Verification items for the finished model (mm, model axes). A direction names the side the tool comes from. Give positions to 0.01 mm unless a question says otherwise; leave off trailing zeros. Loops run counter-clockwise (first coordinate to the right, second up) from the corner with the lowest first, then second, coordinate; pieces in that order, holes last. Notation, with made-up numbers: (77.5, 74.5) -> (85.5, 74.5) arc R8 cw to (85.5, 81.5) -> close; hole circle Ø3 at (61.5, -12). An arc over 180 degrees is marked (long way). Answer in a Markdown table with one row per item. Add a question column.
Q1. Gauge pin test, flat ends, axial feed: P1, Ø12, axis at x = 16.5, y = 27.5, coming from the -Z side; P2, Ø1.8, axis at x = 6.5, z = 3.5, coming from the -Y side. Record the tip position at first contact, or that the pin passes through.
Q2. Material ranges on probe 1 along Y at (x, z) = (10, 4.05); probe 2 along Y at (x, z) = (12, 2.75); probe 3 along X at (y, z) = (32, 2.95), recorded low to high.
Q3. Section check C-C on y = 7. Enter the section's corners in (x, z), and give its area (3 significant figures).
Q4. Section check B-B on z = 2.5. Give the number of separate pieces and of enclosed holes in the cut face, and give its area (3 significant figures).
Q5. Section check A-A on x = 10. Enter the section's corners in (y, z).
Q6. Section check D-D on y = 18.5. Enter the section's corners in (x, z).
Q7. Release check for a two-part mould opening along Y. For faces 1 (the face through (10, 40, 2)), 2 (the face through (13, 0, 2)), 3 (the face through (12.5, 17, 2)), 4 (the face through (0, 18, 2)) record: pulls with the +Y half, pulls with the -Y half, needs draft (parallel to the pull), parting line crosses it, or undercut.
Q8. Set-up check for faces 5 (the face through (12, 3, 2)), 6 (the face through (10, 23, 0)), 7 (the face through (8.5, 8, 2)): record each of +Z, -Z, +X, -X, +Y, -Y from which the full face is reachable in a straight line by a thin tool's end or side.
```python
from build123d import *

# Parameters (mm, degrees)
SKETCH1_R           = 1.5
SKETCH1_W           = 5
SKETCH1_H           = 5
BOSS_EXTRUDE1_DEPTH = 5


with BuildPart() as part:
    # Sketch1 → Boss-Extrude1 (new body)
    with BuildSketch(Plane.XY):
        Polygon((0, 0), (0, 40), (20, 40), (20, 0), (20, -5), (15, -5), (15, 0), (11.5, 0), (11.5, 3), (12.6, 3), (12.6, 5.3), (11.5, 5.3), (11.5, 10), (8.5, 10), (8.5, 5.3), (7.4, 5.3), (7.4, 3), (8.5, 3), (8.5, 0), (5, 0), (5, -5), (0, -5), align=None)
        with Locations((10, 25)):
            Circle(SKETCH1_R, mode=Mode.SUBTRACT)
        with Locations((10, 17.5)):
            Rectangle(SKETCH1_W, SKETCH1_H, mode=Mode.SUBTRACT)
        with Locations((10, 32.5)):
            Rectangle(SKETCH1_W, SKETCH1_H, mode=Mode.SUBTRACT)
    extrude(amount=BOSS_EXTRUDE1_DEPTH)


solid = part.part
```
Taken from the geometry:
| question | item | result |
|---|---|---|
| 1 | P1 | stops at z = 0 |
| 1 | P2 | stops at y = 0 |
| 2 | probe 1 | y = 10 to 15, 20 to 23.5, 26.5 to 30, 35 to 40 |
| 2 | probe 2 | y = 0 to 3, 5.3 to 15, 20 to 30, 35 to 40 |
| 2 | probe 3 | x = 0 to 7.5, 12.5 to 20 |
| 3 | outline | (0, 0) -> (8.5, 0) -> (8.5, 5) -> (0, 5) -> close; (11.5, 0) -> (20, 0) -> (20, 5) -> (11.5, 5) -> close |
| 3 | area | 85.0 mm² |
| 4 | separate pieces | 1 |
| 4 | enclosed holes | 3 |
| 4 | area | 758 mm² |
| 5 | outline | (10, 0) -> (15, 0) -> (15, 5) -> (10, 5) -> close; (20, 0) -> (23.5, 0) -> (23.5, 5) -> (20, 5) -> close; (26.5, 0) -> (30, 0) -> (30, 5) -> (26.5, 5) -> close; (35, 0) -> (40, 0) -> (40, 5) -> (35, 5) -> close |
| 6 | outline | (0, 0) -> (7.5, 0) -> (7.5, 5) -> (0, 5) -> close; (12.5, 0) -> (20, 0) -> (20, 5) -> (12.5, 5) -> close |
| 7 | face 1 | pulls with the +Y half |
| 7 | face 2 | pulls with the -Y half |
| 7 | face 3 | undercut |
| 7 | face 4 | needs draft |
| 8 | face 5 | +Z, -Z |
| 8 | face 6 | -Z, +X, -X, +Y, -Y |
| 8 | face 7 | +Z, -Z, -Y |
